Answer from the drawing. Dimensions are ordinates in mm from the lowest x, y and z of the part. A direction names the side the tool comes from. Give positions to 0.01 mm unless a question says otherwise; leave off trailing zeros. Write each loop counter-clockwise with the first axis right and the second up, starting at its lowest first coordinate (ties: lowest second). Pieces come first, ordered by that corner, then holes. Notation, with made-up numbers: (21.25, -25) - (41.25, -25) arc R31 ccw to (41.25, 0) - close; hole circle Ø3 at (-26, -14). An arc over 180 degrees is marked (long way). Write item = value, one per line.
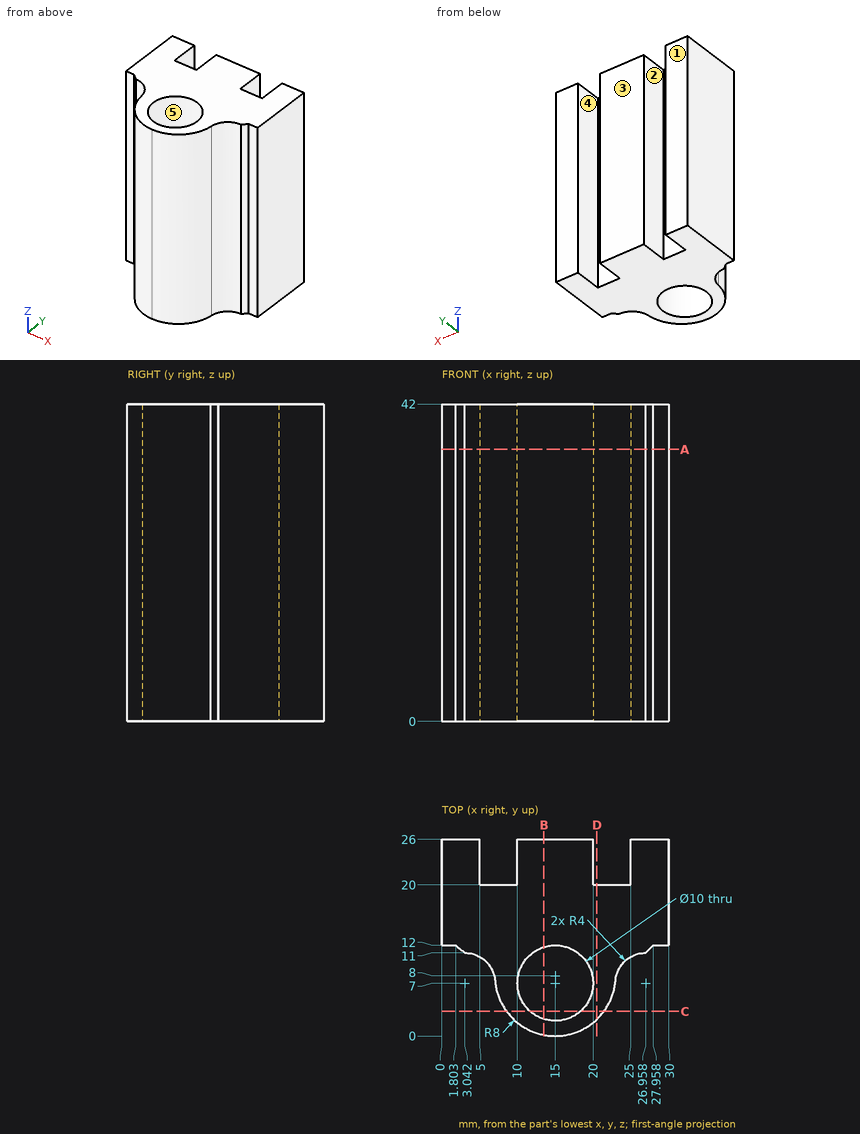
1. A tool of negligible diameter and unlimited length cuts with its end or side. For the marked faces 1 and 2, from which of +Z, -Z, +X, -X, +Y, -Y can it reach the whole face along a straight path? Write none if from no direction.
Solution:
face_1 = +Z, -Z, +X, -X, +Y
face_2 = +Z, -Z, +Y
2. Find section A-A, the plane z = 36. Give the vertices of the cut face in (x, y), then the cut area to 3 significant figures.
Solution:
outline = (0, 12) - (1.8, 12) - (3.04, 11) arc R4 cw to (7.03, 7.33) arc R8 ccw to (22.97, 7.33) arc R4 cw to (26.96, 11) - (27.96, 12) - (30, 12) - (30, 26) - (25, 26) - (25, 20) - (20, 20) - (20, 26) - (10, 26) - (10, 20) - (5, 20) - (5, 26) - (0, 26) - close; hole circle Ø10 at (15, 7)
area = 462 mm^2
3. Given pin 1 (2 mm diameter, centred on x = 1.5, z = 30, fed in from -Y); pin 2 (5 mm diameter, centred on x = 26, y = 6.5, fed in from -Z); pin 3 (0.6 mm diameter, centred on x = 28.5, z = 30, fed in from -Y); pin 4 (1 mm diameter, centred on x = 7, z = 15.5, fed in from +Y), each flat-ended and moving along its own axis, determine where each tip first touches the part or whether it passes through.
Solution:
pin_1 = 11.44
pin_2 = through
pin_3 = 12
pin_4 = 20
4. Find section B-B, the plane x = 13.5. Give the vertices of the cut face in (y, z), then the cut area to 3 significant figures.
Solution:
outline = (0.14, 0) - (2.23, 0) - (2.23, 42) - (0.14, 42) - close; (11.77, 0) - (26, 0) - (26, 42) - (11.77, 42) - close
area = 685 mm^2
5. Find section C-C, the plane y = 3.25. Give the vertices of the cut face in (x, z).
Solution:
outline = (8.56, 0) - (11.69, 0) - (11.69, 42) - (8.56, 42) - close; (18.31, 0) - (21.44, 0) - (21.44, 42) - (18.31, 42) - close
6. For a pull along Y with two mould halves and no side action, classify the marked faces 3, 4 and 5 as pulls with the +Y half, pulls with the -Y half, needs draft (parallel to the pull), parting line crosses it, or undercut.
Solution:
face_3 = pulls with the +Y half
face_4 = needs draft
face_5 = undercut
7. Find section D-D, the plane x = 20.5. Give the vertices of the cut face in (y, z), then the cut area to 3 significant figures.
Solution:
outline = (2.19, 0) - (20, 0) - (20, 42) - (2.19, 42) - close
area = 748 mm^2
8. Straight lines are drawn through the part: line 1 (X direction, y = 20.5, z = 40); line 2 (Y direction, x = 15, z = 15); line 3 (X direction, y = 1.75, z = 5.5) (1 decimal). For each, find the intervals that lie inside material, in ascending order.
Solution:
line_1 = 0 to 5, 10 to 20, 25 to 30
line_2 = 0 to 2, 12 to 26
line_3 = 10 to 20
